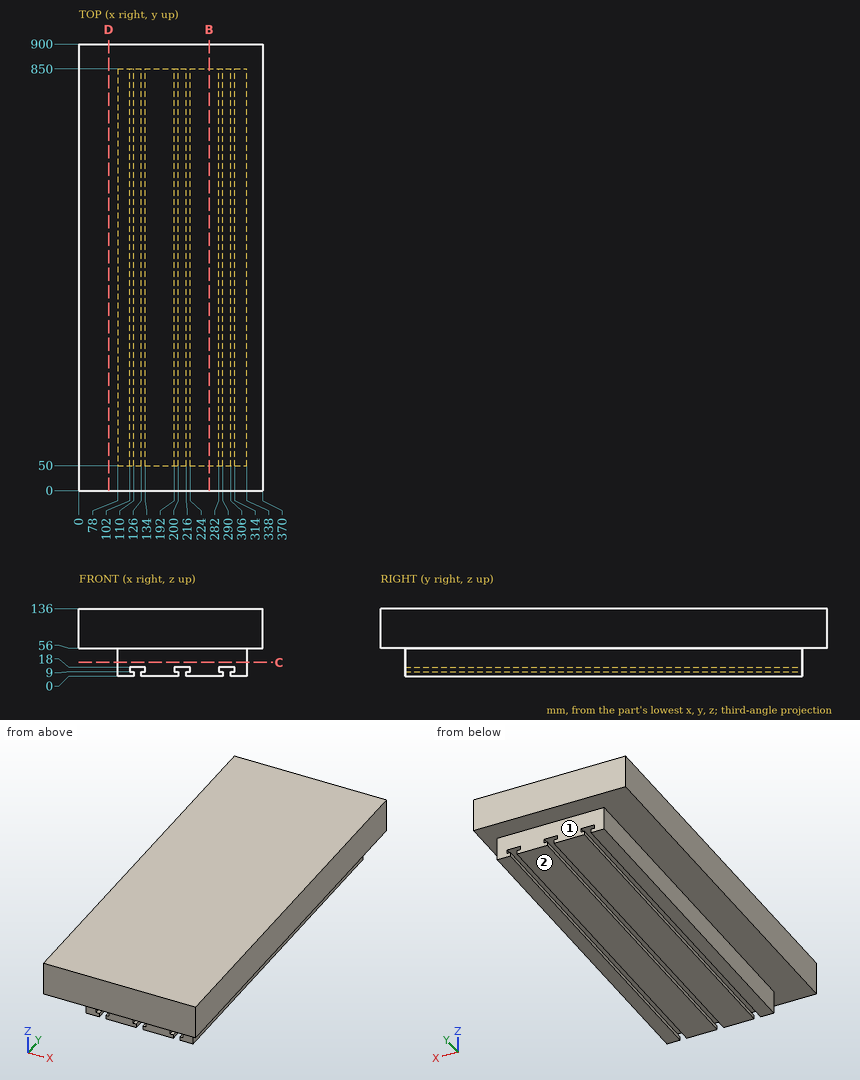
Design review of the part shown in the three views and the two pictorial views. Dimensions are in mm from the part's minimum x, y and z. A direction names the side the tool comes from. Round coordinates to 2 decimals unless told otherwise and drop trailing zeros. Loops run counter-clockwise (first coordinate to the right, second up) from the corner with the lowest first, then second, coordinate; pieces in that order, holes last. Notation, with made-up numbers: M 70.5,45.5 L 85.5,45.5 A17 cw 85.5,72.5 Z; hole C 41,-9 d11. An arc over 180 degrees is marked long. Answer as a JSON object with one key per item and string values.
Item 1: We need section D-D, the plane x = 60. State the section outline as (y, z) points, and give its area (3 significant figures).
Check sheet entries:
{"outline": "M 0,56 L 900,56 L 900,136 L 0,136 Z", "area": "72,000 mm2"}
Item 2: Clearance check with flat-ended pins moving along their axes: P1, Ø10, axis at y = 450.5, z = 13.5, coming from the -X side; P2, Ø6, axis at x = 160, y = 156.5, coming from the -Z side; P3, Ø1.5, axis at y = 332.5, z = 41, coming from the +X side; P4, Ø8, axis at x = 300, y = 795, coming from the -Z side. State where each tip first meets the part, or that it passes through.
Check sheet entries:
{"P1": "x = 78", "P2": "z = 0", "P3": "x = 338", "P4": "z = 18"}
Item 3: Tool access review of the marked faces 1 and 2: name each direction out of +Z, -Z, +X, -X, +Y, -Y from which nothing blocks a thin tool from reaching the whole face with its end or side.
Check sheet entries:
{"face 1": "-Z, +X, -X, +Y", "face 2": "-Z, +X, -X, +Y, -Y"}
Item 4: For line 1 along X through (y, z) = (525, 13.5); line 2 along Z through (x, y) = (285, 507.5); line 3 along Z through (x, y) = (38.5, 511.5), list the stretches that pass through material, from the lowest coordinate up.
Check sheet entries:
{"line 1": "78 to 102, 134 to 192, 224 to 282, 314 to 338", "line 2": "0 to 9, 18 to 136", "line 3": "56 to 136"}
Item 5: We need section B-B, the plane x = 262.5. State the section outline as (y, z) points, and give its area (3 significant figures).
Check sheet entries:
{"outline": "M 0,56 L 50,56 L 50,0 L 850,0 L 850,56 L 900,56 L 900,136 L 0,136 Z", "area": "117,000 mm2"}
Item 6: We need section C-C, the plane z = 27.5. State the section outline as (x, y) points, and give its area (3 significant figures).
Check sheet entries:
{"outline": "M 78,50 L 338,50 L 338,850 L 78,850 Z", "area": "208,000 mm2"}
